Part print with two shaded views. Sizes in mm from the minimum x, y, z corner. Give positions to 0.01 mm unless a question says otherwise; leave off trailing zeros. Order: outer loops, then holes, each group sorted by start corner. A loop starts at its lowest first (then second) coordinate and runs counter-clockwise, first axis right, second up. Notation, with made-up numbers: M 11.25,61 L 23.25,61 A10 ccw 23.25,73 Z; hole C 3,-12 d2. An arc over 180 degrees is marked long. Answer as CSV lines item,"result".
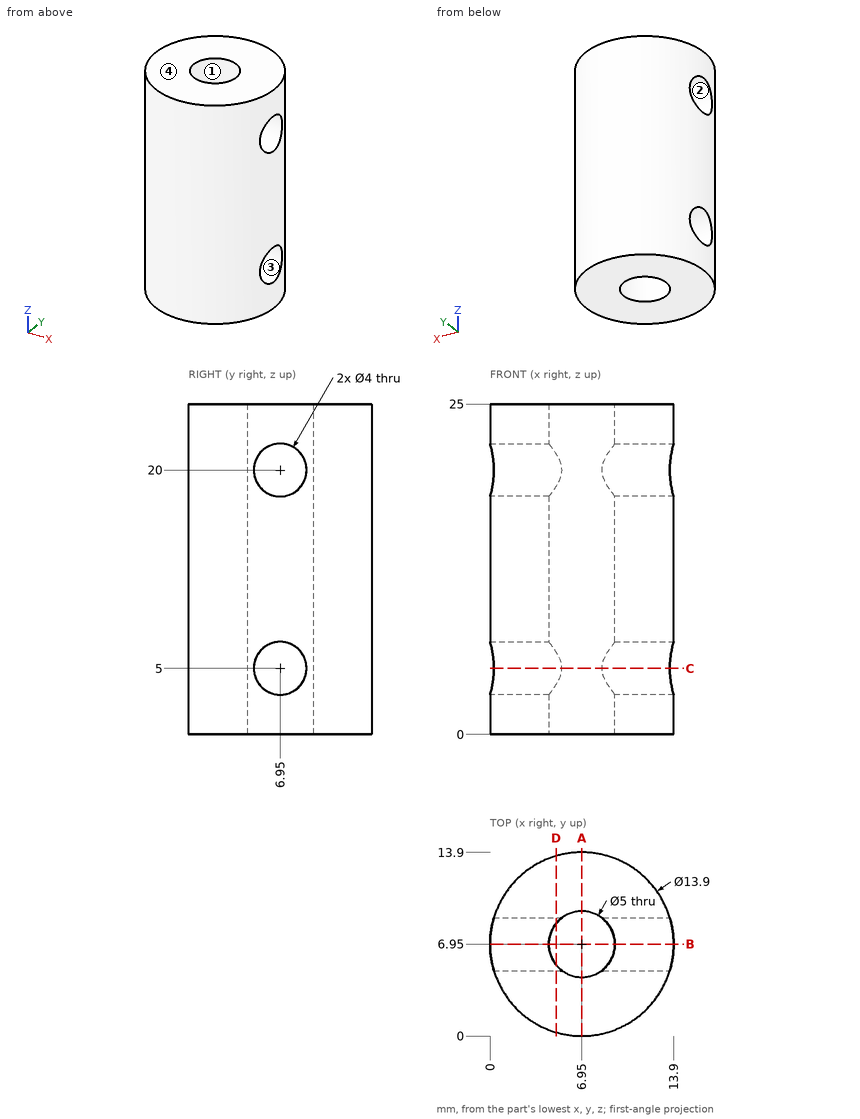
Item 1: Pull direction Z, two halves, no side cores. Call the marked faces 1, 2, 3 and 4: released by +Z, released by -Z, zero draft, split by the parting line, or undercut.
Geometry says:
face 1,"zero draft"
face 2,"undercut"
face 3,"undercut"
face 4,"released by +Z"
Item 2: Band-saw the part on B-B (y = 6.95). Give the cut face in (x, z).
Geometry says:
outline,"M 0,0 L 4.45,0 L 4.45,3 L 0,3 Z; M 0,7 L 4.45,7 L 4.45,18 L 0,18 Z; M 0,22 L 4.45,22 L 4.45,25 L 0,25 Z; M 9.45,0 L 13.9,0 L 13.9,3 L 9.45,3 Z; M 9.45,7 L 13.9,7 L 13.9,18 L 9.45,18 Z; M 9.45,22 L 13.9,22 L 13.9,25 L 9.45,25 Z"
Item 3: Probe line 1 along Y through (x, z) = (6.95, 6.25); line 2 along Z through (x, y) = (10, 5.25); line 3 along Y through (x, z) = (9.75, 4.75). List the from-to ranges inside material, lowest first. Write a range as from..to.
Geometry says:
line 1,"y = 0..4.45, 9.45..13.9"
line 2,"z = 0..3.95, 6.05..18.95, 21.05..25"
line 3,"y = 0.59..4.97, 8.93..13.31"
Item 4: Band-saw the part on D-D (x = 5). Give the cut face in (y, z).
Geometry says:
outline,"M 0.28,0 L 5.39,0 L 5.39,3.75 A2 cw 5.39,6.25 L 5.39,18.75 A2 cw 5.39,21.25 L 5.39,25 L 0.28,25 Z; M 8.51,0 L 13.62,0 L 13.62,25 L 8.51,25 L 8.51,21.25 A2 cw 8.51,18.75 L 8.51,6.25 A2 cw 8.51,3.75 Z"
Item 5: Band-saw the part on A-A (x = 6.95). Give the cut face in (y, z), and give its area (4 significant figures).
Geometry says:
outline,"M 0,0 L 4.45,0 L 4.45,25 L 0,25 Z; M 9.45,0 L 13.9,0 L 13.9,25 L 9.45,25 Z"
area,"222.5 mm2"
Item 6: Drop flat-ended pins along their axis: pin 1 (1.5 mm diameter, centred on x = 2.5, z = 7, fed in from -Y); pin 2 (1.5 mm diameter, centred on y = 3, z = 16.5, fed in from +X); pin 3 (3 mm diameter, centred on x = 12, z = 18.5, fed in from -Y). Give the stop position or say it passes through.
Geometry says:
pin 1,"stops at y = 1.07"
pin 2,"stops at x = 13.12"
pin 3,"stops at y = 0.98"
Item 7: Band-saw the part on C-C (z = 5). Give the cut face in (x, y).
Geometry says:
outline,"M 0.29,4.95 A6.95 ccw 13.61,4.95 L 8.45,4.95 A2.5 cw 5.45,4.95 Z; M 0.29,8.95 L 5.45,8.95 A2.5 cw 8.45,8.95 L 13.61,8.95 A6.95 ccw Z"
